```python
from build123d import *

# Parameters (mm, degrees)
SKETCH1_R           = 27.5
BOSS_EXTRUDE1_DEPTH = 317.215559
SKETCH2_R           = 19.658611568
CUT_EXTRUDE1_DEPTH  = 320.590692718
CHAMFER1_SIZE       = 5.390289
CHAMFER1_SIZE_2     = 9.336255


with BuildPart() as part:
    # Sketch1 → Boss-Extrude1 (new body)
    with BuildSketch(Plane(origin=(0, 0, 0), x_dir=(1, 0, 0), z_dir=(0, 1, 0))):
        with Locations(Location((0, 0, 0), (0, 0, 270))):
            Circle(SKETCH1_R)
    extrude(amount=BOSS_EXTRUDE1_DEPTH)

    # Sketch2 → Cut-Extrude1 (cut, through all)
    with BuildSketch(Plane(origin=(0, 0, 0), x_dir=(1, 0, 0), z_dir=(0, 1, 0))):
        with Locations(Location((0, 0, 0), (0, 0, 270))):
            Circle(SKETCH2_R)
    extrude(amount=CUT_EXTRUDE1_DEPTH, mode=Mode.SUBTRACT)

    # Chamfer1
    # the kernel refuses this chamfer: 9.336255, 5.390289 mm, written as the material it takes off along each edge
    with BuildSketch(Plane(origin=(0, 317.215559, 0), x_dir=(0, 0, 1), z_dir=(-1, 0, 0))) as chamfer1_piece_1:
        Polygon((27.5, -CHAMFER1_SIZE), (27.5 - CHAMFER1_SIZE_2, 0), (27.5, 0), align=None)
    revolve(axis=Axis((0, 317.215559, 0), (0, 1, 0)), mode=Mode.SUBTRACT)
    with BuildSketch(Plane(origin=(0, 0, 0), x_dir=(0, 0, 1), z_dir=(-1, 0, 0))) as chamfer1_piece_2:
        Polygon((27.5, CHAMFER1_SIZE_2), (27.5 - CHAMFER1_SIZE, 0), (27.5, 0), align=None)
    revolve(axis=Axis((0, 0, 0), (0, 1, 0)), mode=Mode.SUBTRACT)


solid = part.part
```
Here's how the part is built. I have some questions about the finished solid (model axes, mm). Round coordinates to 2 decimals unless told otherwise and drop trailing zeros. Order: outer loops, then holes, each group sorted by start corner. A loop starts at its lowest first (then second) coordinate and runs counter-clockwise, first axis right, second up. Notation, with made-up numbers: M 44.25,-36 L 82.25,-36 A35 cw 82.25,3 Z; hole C 66.25,83.25 d7. An arc over 180 degrees is marked long. Use CSV: the item, a comma, the result in double quotes.
1) I want a section at B-B (x = 0). List the corners of the cut face in (y, z) for me, then the cut area to 3 significant figures.
Taken from the geometry:
outline,"M 0,-22.11 L 9.34,-27.5 L 311.83,-27.5 L 316.35,-19.66 L 0,-19.66 Z; M 0,19.66 L 316.35,19.66 L 311.83,27.5 L 9.34,27.5 L 0,22.11 Z"
area,"4,880 mm^2"
2) If we mould it in two halves opening along X, with no side actions, what happens to faces 1 (the cylindrical face through (5.905, 155.962, 18.751)), 2 (the conical face through (6.72, 0.453, 21.338)), 3 (the flat face through (-13, 0, -15))? For each: pulls with the +X half, pulls with the -X half, needs draft (parallel to the pull), parting line crosses it, or undercut.
Taken from the geometry:
face 1,"undercut"
face 2,"parting line crosses it"
face 3,"needs draft"
3) I need wall thicknesses on line 1 along X through (y, z) = (205, 0); line 2 along X through (y, z) = (38, -11); line 3 along Z through (x, y) = (2, 262). Which ranges of each line are inside material? Lowest first, please. Write a range as [from, to].
Taken from the geometry:
line 1,"[-27.5, -19.66], [19.66, 27.5]"
line 2,"[-25.2, -16.29], [16.29, 25.2]"
line 3,"[-27.43, -19.56], [19.56, 27.43]"
4) I want a section at A-A (z = 0). List the corners of the cut face in (x, y) for me.
Taken from the geometry:
outline,"M -27.5,9.34 L -22.11,0 L -19.66,0 L -19.66,316.35 L -27.5,311.83 Z; M 19.66,0 L 22.11,0 L 27.5,9.34 L 27.5,311.83 L 19.66,316.35 Z"
5) I want a section at C-C (y = 289). List the corners of the cut face in (x, z) for me, then the cut area to 3 significant figures.
Taken from the geometry:
outline,"C 0,0 d55; hole C 0,0 d39.32"
area,"1,160 mm^2"
6) I'm going to push flat-ended pins straight in: P1, Ø1.5, axis at y = 157, z = 10, coming from the -X side; P2, Ø1.5, axis at y = 55, z = -5.5, coming from the +X side; P3, Ø2, axis at y = 246, z = 10.5, coming from the +X side. Where does each tip first touch, or does it pass through?
Taken from the geometry:
P1,"x = -25.9"
P2,"x = 27.09"
P3,"x = 25.81"
